Verification items for the finished model (mm, model axes). Face numbers are marked on the shaded views. A direction names the side the tool comes from. Coordinates: 2 decimals unless noted, no trailing zeros. Loops run counter-clockwise (first coordinate to the right, second up) from the corner with the lowest first, then second, coordinate; pieces in that order, holes last. Notation, with made-up numbers: (14.5, 75.25) -> (39.5, 75.25) arc R31 cw to (39.5, 101.25) -> close; hole circle Ø1 at (-11, 79.5). An arc over 180 degrees is marked (long way). Answer as a JSON object with one key per item and string values. Group by question number.
Q1. Cross-section at A-A on x = 11.5. Record the boundary of the cut face in (y, z) (3 decimals), and give its area (3 significant figures).
Q2. Cross-section at C-C on x = 18.5. Record the boundary of the cut face in (y, z) (3 decimals).
Q3. Release check for a two-part mould opening along Z. For the marked faces 3, 4, 5 and 6 record: released by +Z, released by -Z, zero draft, split by the parting line, or undercut.
Q4. Set-up check for the marked faces 1 and 2: record each of +Z, -Z, +X, -X, +Y, -Y from which the full face is reachable in a straight line by a thin tool's end or side.
Q5. Scan lines: L1, parallel to Y at x = 0, z = 32.15 (3 decimals); L2, parallel to Z at x = 2, y = 1; L3, parallel to Z at x = 15.5, y = -1.25. Record each from-to range of solid material in increasing order.
Q6. Gauge pin test, flat ends, axial feed: pin 1 Ø3 at (x, y) = (8.5, 0.5) entering from -Z; pin 2 Ø6 at (x, z) = (18, 14) entering from +Y; pin 3 Ø3.5 at (y, z) = (0.5, 16) entering from -X. Record the tip position at first contact, or that the pin passes through.
```python
from build123d import *

# Parameters (mm, degrees)
BOSS_EXTRUDE10_DEPTH = 2
BOSS_EXTRUDE15_DEPTH = 1.5
BOSS_EXTRUDE17_START = 2
SKETCH1_17_W         = 29.75
SKETCH1_17_H         = 3
BOSS_EXTRUDE17_DEPTH = 35.2
SKETCH2_W            = 23.8
SKETCH2_H            = 5
BOSS_EXTRUDE18_DEPTH = 1.5
FILLET1_R            = 2
FILLET3_R            = 2
FILLET2_R            = 3.375
FILLET5_R            = 2.5
SKETCH4_R            = 1.85
BOSS_EXTRUDE19_DEPTH = 1.5
FILLET4_R            = 1.5


# Some blends are built 0.0001 mm under size
with BuildPart() as part:
    # Sketch1 → Boss-Extrude10 (new body)
    # profile 1 of 6: a face of its own
    with BuildSketch(Plane.XY.offset(33.2)):
        Polygon((-4.25, 3.375), (-4.25, -3.375), (19.5, -3.375), (19.5, -1.5), (19.5, 1.5), (19.5, 3.375), align=None)
        with BuildLine():
            ThreePointArc((2.515308132, -1.635), (-2.636759375, -1.430908802), (0, 3))
            ThreePointArc((0, 3), (1.430908802, 2.636759375), (2.515308132, 1.635))
            Line((2.515308132, 1.635), (12.065, 1.635))
            ThreePointArc((12.065, 1.635), (13.7, 0), (12.065, -1.635))
            Line((12.065, -1.635), (2.515308132, -1.635))
        make_face(mode=Mode.SUBTRACT)
    # profile 2 of 6: a face of its own
    with BuildSketch(Plane.XY.offset(33.2)):
        with BuildLine():
            Line((12.065, 1.635), (2.515308132, 1.635))
            ThreePointArc((2.515308132, 1.635), (2.876275751, 0.852665117), (3, 0))
            ThreePointArc((3, 0), (2.876275751, -0.852665117), (2.515308132, -1.635))
            Line((2.515308132, -1.635), (12.065, -1.635))
            Line((12.065, -1.635), (12.065, 1.635))
        make_face()
    # profile 3 of 6: a face of its own
    with BuildSketch(Plane.XY.offset(33.2)):
        with BuildLine():
            ThreePointArc((12.065, 1.635), (13.7, 0), (12.065, -1.635))
            Line((12.065, -1.635), (12.065, 1.635))
        make_face()
    # profile 4 of 6: a face of its own
    with BuildSketch(Plane.XY.offset(33.2)):
        with BuildLine():
            Line((0, 1.125), (0, 1.635))
            Line((0, 1.635), (0, 3))
            ThreePointArc((0, 3), (-2.636759375, -1.430908802), (2.515308132, -1.635))
            Line((2.515308132, -1.635), (0, -1.635))
            Line((0, -1.635), (0, -1.125))
            ThreePointArc((0, -1.125), (-1.125, 0), (0, 1.125))
        make_face()
    # profile 5 of 6: a face of its own
    with BuildSketch(Plane.XY.offset(33.2)):
        with BuildLine():
            Line((2.515308132, 1.635), (0, 1.635))
            Line((0, 1.635), (0, 1.125))
            ThreePointArc((0, 1.125), (0.795495129, 0.795495129), (1.125, 0))
            ThreePointArc((1.125, 0), (0.795495129, -0.795495129), (0, -1.125))
            Line((0, -1.125), (0, -1.635))
            Line((0, -1.635), (2.515308132, -1.635))
            ThreePointArc((2.515308132, -1.635), (2.876275751, -0.852665117), (3, 0))
            ThreePointArc((3, 0), (2.876275751, 0.852665117), (2.515308132, 1.635))
        make_face()
    # profile 6 of 6: a face of its own
    with BuildSketch(Plane.XY.offset(33.2)):
        with BuildLine():
            Line((0, 3), (0, 1.635))
            Line((0, 1.635), (2.515308132, 1.635))
            ThreePointArc((2.515308132, 1.635), (1.430908802, 2.636759375), (0, 3))
        make_face()
    extrude(amount=BOSS_EXTRUDE10_DEPTH)

    # Sketch1<16> → Boss-Extrude15 (add)
    with BuildSketch(Plane.XY.offset(33.2)):
        Polygon((-4.25, 3.375), (-4.25, -3.375), (19.5, -3.375), (19.5, -1.5), (19.5, 1.5), (19.5, 3.375), align=None)
        with BuildLine():
            ThreePointArc((12.065, 1.635), (13.7, 0), (12.065, -1.635))
            Line((12.065, -1.635), (2.515308132, -1.635))
            ThreePointArc((2.515308132, -1.635), (-3, 0), (2.515308132, 1.635))
            Line((2.515308132, 1.635), (12.065, 1.635))
        make_face(mode=Mode.SUBTRACT)
    extrude(amount=-BOSS_EXTRUDE15_DEPTH)

    # Sketch1<17> → Boss-Extrude17 (add)
    with BuildSketch(Plane.XY.offset(33.2).offset(BOSS_EXTRUDE17_START)):
        with Locations((34.375, 0)):
            Rectangle(SKETCH1_17_W, SKETCH1_17_H)
    extrude(amount=-BOSS_EXTRUDE17_DEPTH)

    # Sketch2 → Boss-Extrude18 (add)
    with BuildSketch(Plane(origin=(0, 0, 0), x_dir=(-1, 0, 0), z_dir=(0, 0, -1))):
        with Locations((-7.6, 0)):
            Rectangle(SKETCH2_W, SKETCH2_H)
    extrude(amount=-BOSS_EXTRUDE18_DEPTH)

    # Fillet1
    # the kernel refuses this fillet: 2 mm, written as the material it adds along each edge
    with BuildSketch(Plane(origin=(19.5, 1.5, 1.5), x_dir=(1, 0, 0), z_dir=(0, 0, -1))) as fillet1_piece_1:
        with BuildLine():
            CenterArc((1.732050808, -2), FILLET1_R, 90, 60)
            Line((0, -1), (0, 0))
            Line((0, 0), (1.732050808, 0))
        make_face()
    extrude(amount=1.5)
    with BuildSketch(Plane(origin=(19.5, -1.5, 1.5), x_dir=(1, 0, 0), z_dir=(0, 0, -1))) as fillet1_piece_2:
        with BuildLine():
            CenterArc((1.732050808, 2), FILLET1_R, 210, 60)
            Line((0, 1), (0, 0))
            Line((0, 0), (1.732050808, 0))
        make_face()
    extrude(amount=1.5)
    with BuildSketch(Plane(origin=(19.5, -1.5, 35.2), x_dir=(0, -1, 0), z_dir=(0, 0, -1))) as fillet1_piece_3:
        with BuildLine():
            CenterArc((2, -1.996089928), FILLET1_R, 93.583321698, 86.416678302)
            Line((0, -1.996089928), (0, 0))
            Line((0, 0), (1.875, 0))
        make_face()
    extrude(amount=3.5)
    with BuildSketch(Plane(origin=(19.5, 1.5, 35.2), x_dir=(0, 1, 0), z_dir=(0, 0, -1))) as fillet1_piece_4:
        with BuildLine():
            CenterArc((2, 1.996089928), FILLET1_R, 180, 86.416678302)
            Line((0, 1.996089928), (0, 0))
            Line((0, 0), (1.875, 0))
        make_face()
    extrude(amount=3.5)

    # Fillet3
    fillet3_edges = [part.edges().sort_by_distance(p)[0] for p in [
        (19.5, 0, 31.7),
        (19.5, 0, 1.5),
    ]]
    fillet(fillet3_edges, radius=FILLET3_R)

    # Fillet2
    fillet2_edges = [part.edges().sort_by_distance(p)[0] for p in [
        (-4.25, 3.375, 33.45),
        (-4.25, -3.375, 33.45),
    ]]
    fillet(fillet2_edges, radius=FILLET2_R - 0.0001)  # a hair under: the kernel refuses the full size

    # Fillet5
    fillet5_edges = [part.edges().sort_by_distance(p)[0] for p in [
        (-4.3, -2.5, 0.75),
        (-4.3, 2.5, 0.75),
    ]]
    fillet(fillet5_edges, radius=FILLET5_R - 0.0001)  # a hair under: the kernel refuses the full size

    # Sketch4 → Boss-Extrude19 (add)
    with BuildSketch(Plane(origin=(0, 0, 0), x_dir=(-1, 0, 0), z_dir=(0, 0, -1))):
        with Locations(Location((0, 0, 0), (0, 0, 180))):
            Circle(SKETCH4_R)
    extrude(amount=BOSS_EXTRUDE19_DEPTH)

    # Fillet4
    fillet4_edges = [part.edges().sort_by_distance(p)[0] for p in [
        (49.25, 1.5, 17.6),
        (49.25, -1.5, 17.6),
    ]]
    fillet(fillet4_edges, radius=FILLET4_R - 0.0001)  # a hair under: the kernel refuses the full size


solid = part.part
```
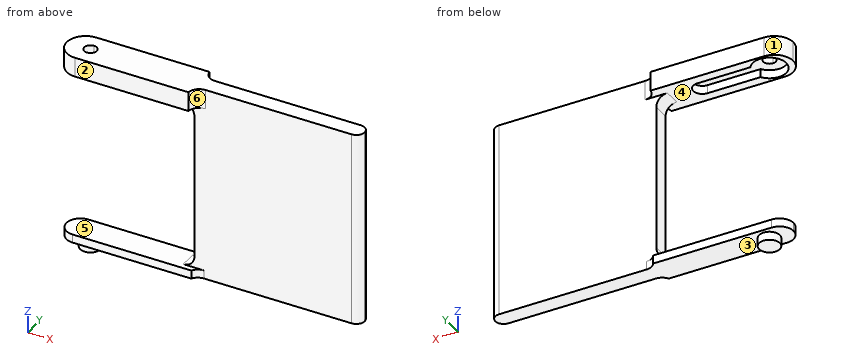
Computed values:
{
 "1": {"outline": "(-3.375, 31.7) -> (-1.635, 31.7) -> (-1.635, 33.2) -> (1.635, 33.2) -> (1.635, 31.7) -> (3.375, 31.7) -> (3.375, 35.2) -> (-3.375, 35.2) -> close; (-2.5, 0) -> (2.5, 0) -> (2.5, 1.5) -> (-2.5, 1.5) -> close", "area": "26.2 mm²"},
 "2": {"outline": "(-3.375, 31.7) -> (-1.5, 31.7) -> (-1.5, 31.432) -> (1.5, 31.432) -> (1.5, 31.7) -> (3.375, 31.7) -> (3.375, 35.2) -> (-3.375, 35.2) -> close; (-2.5, 0) -> (2.5, 0) -> (2.5, 1.5) -> (1.5, 1.5) -> (1.5, 1.768) -> (-1.5, 1.768) -> (-1.5, 1.5) -> (-2.5, 1.5) -> close"},
 "3": {"face 3": "released by -Z", "face 4": "undercut", "face 5": "undercut", "face 6": "zero draft"},
 "4": {"face 1": "+Z, -X, +Y", "face 2": "+Z, -Z, +X, -X, -Y"},
 "5": {"L1": "y = -3.375 to -3, 3 to 3.375", "L2": "z = 0 to 1.5, 33.2 to 35.2", "L3": "z = 0 to 1.5, 31.7 to 35.2"},
 "6": {"pin 1": "stops at z = 0", "pin 2": "stops at y = 1.5", "pin 3": "stops at x = 19.5"}
}
